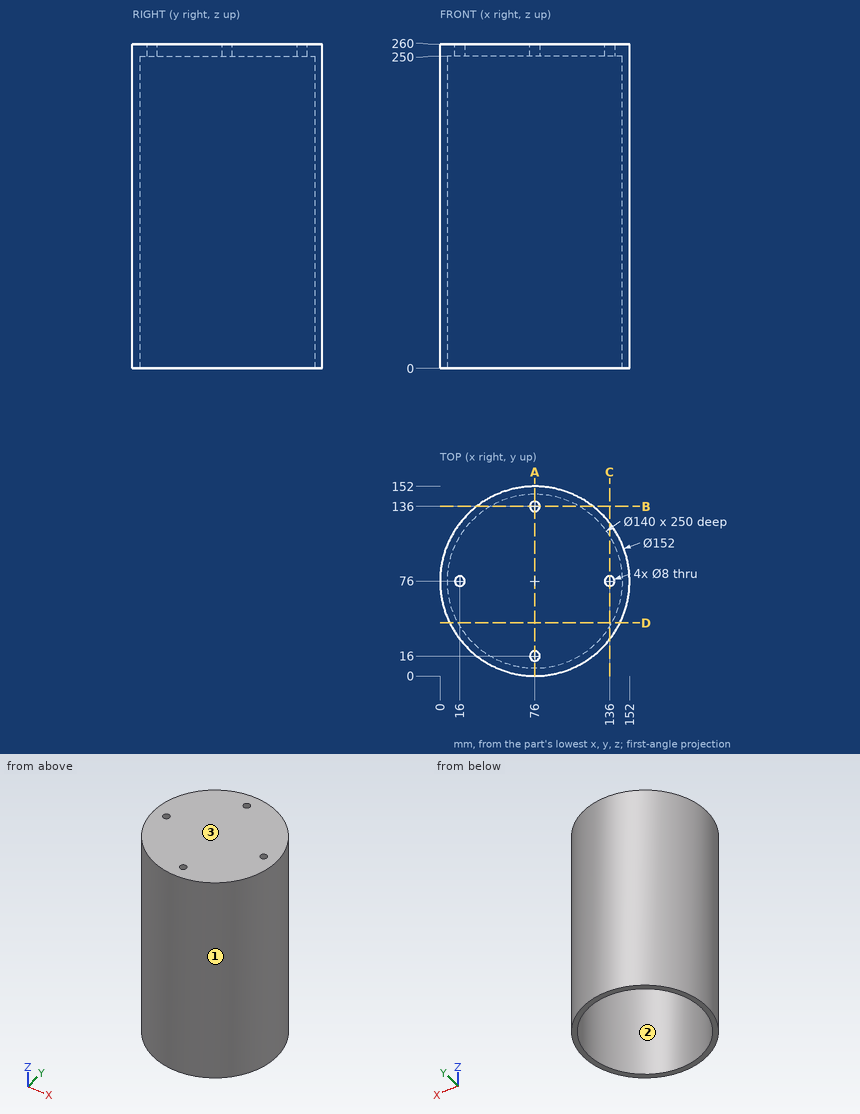
Verification items for this drawing (mm, ordinates from the low corner). Coordinates: 2 decimals unless noted, no trailing zeros. Order: outer loops, then holes, each group sorted by start corner. A loop starts at its lowest first (then second) coordinate and runs counter-clockwise, first axis right, second up. Notation, with made-up numbers: (-26, 13) -> (12, 13) arc R17 ccw to (12, 22) -> close; hole circle Ø8 at (58, 28). An arc over 180 degrees is marked (long way). Put each result on its own line as item: value. Start each with the question number.
1. Cross-section at B-B, the plane y = 136. Record the boundary of the cut face in (x, z), then the cut area to 3 significant figures.
2. Cross-section at A-A, the plane x = 76. Record the boundary of the cut face in (y, z), then the cut area to 3 significant figures.
3. Material ranges on L1, parallel to Y at x = 76, z = 253; L2, parallel to X at y = 78, z = 247; L3, parallel to Y at x = 62, z = 74, recorded low to high. Write a range as [from, to].
4. Go/stop test with flat-tipped pins: pin 1 Ø12 at (y, z) = (29.5, 125) entering from +X; pin 2 Ø1 at (y, z) = (28, 67) entering from -X; pin 3 Ø5 at (y, z) = (80.5, 162) entering from +X. Record where each tip stops, or that it passes through.
5. Cross-section at D-D, the plane y = 42.5. Record the boundary of the cut face in (x, z).
6. Mould release check, pull along X, two halves, no side actions. Record for the marked faces 1, 2 and 3: released by +X, released by -X, zero draft, split by the parting line, or undercut.
Computed:
1. outline: (29.35, 0) -> (39.94, 0) -> (39.94, 250) -> (72, 250) -> (72, 260) -> (29.35, 260) -> close; (80, 250) -> (112.06, 250) -> (112.06, 0) -> (122.65, 0) -> (122.65, 260) -> (80, 260) -> close
1. area: 6,150 mm2
2. outline: (0, 0) -> (6, 0) -> (6, 250) -> (12, 250) -> (12, 260) -> (0, 260) -> close; (20, 250) -> (132, 250) -> (132, 260) -> (20, 260) -> close; (140, 250) -> (146, 250) -> (146, 0) -> (152, 0) -> (152, 260) -> (140, 260) -> close
2. area: 4,360 mm2
3. L1: [0, 12], [20, 132], [140, 152]
3. L2: [0.03, 6.03], [145.97, 151.97]
3. L3: [1.3, 7.41], [144.59, 150.7]
4. pin 1: x = 140.31
4. pin 2: x = 16.67
4. pin 3: x = 151.97
5. outline: (7.78, 0) -> (14.54, 0) -> (14.54, 250) -> (137.46, 250) -> (137.46, 0) -> (144.22, 0) -> (144.22, 260) -> (7.78, 260) -> close
6. face 1: split by the parting line
6. face 2: undercut
6. face 3: zero draft
